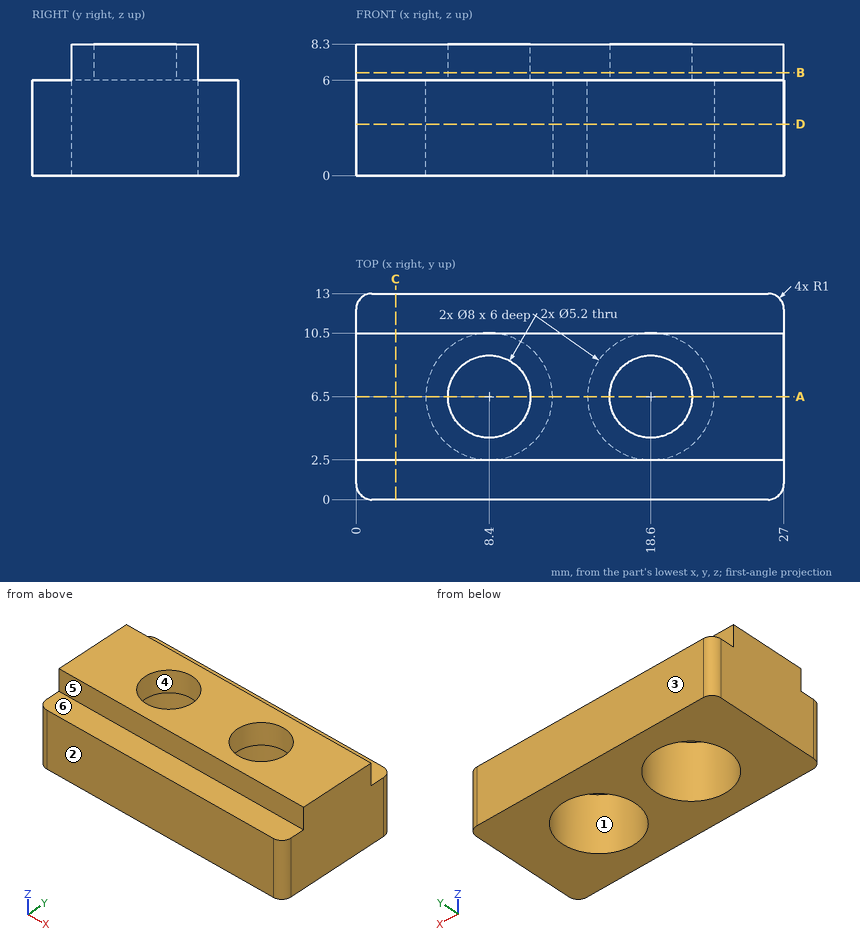
Answer from the drawing. Dimensions are ordinates in mm from the lowest x, y and z of the part. A direction names the side the tool comes from. Give positions to 0.01 mm unless a question says otherwise; leave off trailing zeros. Order: outer loops, then holes, each group sorted by start corner. A loop starts at its lowest first (then second) coordinate and runs counter-clockwise, first axis right, second up. Notation, with made-up numbers: (-9.75, 67) -> (17.25, 67) arc R21 ccw to (17.25, 90) -> close; hole circle Ø2 at (69, 12.25). An arc over 180 degrees is marked (long way). One line per item, written item: value. Start each with the question number.
(1) The part is cut by section A-A (y = 6.5). Determine the outline of the cut face in (x, z).
(2) The part is cut by section B-B (z = 6.5). Determine the outline of the cut face in (x, y), and give its area (3 significant figures).
(3) For a pull along Y with two mould halves and no side action, classify the marked faces 3, 4, 5 and 6 as released by +Y, released by -Y, zero draft, split by the parting line, or undercut.
(4) Straight lines are drawn through the part: L1, parallel to X at y = 3.75, z = 1.5; L2, parallel to X at y = 5.5, z = 4; L3, parallel to Y at x = 18.6, z = 4.45. For each, find the intervals that lie inside material, in ascending order.
(5) Flat-ended cylindrical pins translate along their axes: P1, Ø2.5, axis at x = 10, y = 8, coming from the -Z side; P2, Ø1.2, axis at x = 7, z = 7, coming from the +Y side; P3, Ø1.3, axis at x = 7.5, y = 1.5, coming from the +Z side. Find the tip coordinate at first contact, or state that the pin passes through.
(6) The part is cut by section C-C (x = 2.5). Determine the outline of the cut face in (y, z), and give its area (3 significant figures).
(7) A tool of negligible diameter and unlimited length cuts with its end or side. For the marked faces 1 and 2, from which of +Z, -Z, +X, -X, +Y, -Y can it reach the whole face along a straight path? Write none if from no direction.
(8) The part is cut by section D-D (z = 3.25). Determine the outline of the cut face in (x, y).
Taken from the geometry:
1. outline: (0, 0) -> (4.4, 0) -> (4.4, 6) -> (5.8, 6) -> (5.8, 8.3) -> (0, 8.3) -> close; (11, 6) -> (12.4, 6) -> (12.4, 0) -> (14.6, 0) -> (14.6, 6) -> (16, 6) -> (16, 8.3) -> (11, 8.3) -> close; (21.2, 6) -> (22.6, 6) -> (22.6, 0) -> (27, 0) -> (27, 8.3) -> (21.2, 8.3) -> close
2. outline: (0, 2.5) -> (27, 2.5) -> (27, 10.5) -> (0, 10.5) -> close; hole circle Ø5.2 at (8.4, 6.5); hole circle Ø5.2 at (18.6, 6.5)
2. area: 174 mm^2
3. face 3: released by +Y
3. face 4: undercut
3. face 5: released by -Y
3. face 6: zero draft
4. L1: 0 to 5.5, 11.3 to 15.7, 21.5 to 27
4. L2: 0 to 4.53, 12.27 to 14.73, 22.47 to 27
4. L3: 0 to 2.5, 10.5 to 13
5. P1: z = 6
5. P2: y = 10.5
5. P3: z = 6
6. outline: (0, 0) -> (13, 0) -> (13, 6) -> (10.5, 6) -> (10.5, 8.3) -> (2.5, 8.3) -> (2.5, 6) -> (0, 6) -> close
6. area: 96.4 mm^2
7. face 1: -Z
7. face 2: +Z, -Z, +X, -X, -Y
8. outline: (0, 1) arc R1 ccw to (1, 0) -> (26, 0) arc R1 ccw to (27, 1) -> (27, 12) arc R1 ccw to (26, 13) -> (1, 13) arc R1 ccw to (0, 12) -> close; hole circle Ø8 at (8.4, 6.5); hole circle Ø8 at (18.6, 6.5)
